Work out the finished part from the listing and answer in its coordinate system (mm). A direction names the side the tool comes from. Coordinates: 2 decimals unless noted, no trailing zeros. Write each loop counter-clockwise with the first axis right and the second up, starting at its lowest first coordinate (ties: lowest second). Pieces come first, ordered by that corner, then holes. Notation, with made-up numbers: M -29.75,84 L -13.75,84 A16 ccw -13.75,107 Z; hole C 31.25,-16.5 d6. An arc over 180 degrees is marked long. Answer as CSV lines item,"result". Start each with the question number.
(1) The mould has two halves that part along Y. Classify faces 1 (the flat face through (10, -4, 7)), 2 (the flat face through (0, -5, 7)), 3 (the cylindrical face through (4.991, 2.123, 7.395)), 4 (the cylindrical face through (-14.991, 2.123, 7.395)): released by +Y, released by -Y, zero draft, split by the parting line, or undercut.
(2) A cutting plane is placed at A-A on x = 2.5. Give the vertices of the cut face in (y, z).
(3) A cutting plane is placed at D-D on x = -17.5. Give the vertices of the cut face in (y, z), then the cut area to 3 significant figures.
(4) Flat-ended cylindrical pins translate along their axes: P1, Ø1.5, axis at y = -1, z = 3, coming from the -X side; P2, Ø3, axis at y = 4, z = 4.5, coming from the -X side; P3, Ø1, axis at x = -13.5, z = 4, coming from the -Y side. Find the tip coordinate at first contact, or state that the pin passes through.
(5) Find the intervals of material crossed by L1, parallel to Y at x = 2.5, z = 7.5; L2, parallel to Y at x = 5, z = 9; L3, parallel to X at y = -4, z = 1, in increasing order. Write a range as [from, to].
(6) For faces 5 (the cylindrical face through (7.6, -3, 7.4)), 6 (the flat face through (-10, 4, 7)), 7 (the flat face through (-5, 0, 0)), 8 (the flat face through (10, 4, 7)), 9 (the flat face through (-10, -4, 7)), determine the directions among +Z, -Z, +X, -X, +Y, -Y from which every point of the face is accessible in a straight line to the end or side of a thin tool.
(7) A cutting plane is placed at C-C on y = 0. Give the vertices of the cut face in (x, z), then the cut area to 3 significant figures.
(8) A cutting plane is placed at B-B on z = 8.5. Give the vertices of the cut face in (x, y) (1 decimal).
from build123d import *

# Parameters (mm, degrees)
F1_DEPTH = 15


with BuildPart() as f1:
    # F0 (on Top) → F1 (new body)
    with BuildSketch(Plane.XY):
        with BuildLine():
            Line((-10, -5), (10, -5))
            Line((10, -5), (10, -2.459675))
            ThreePointArc((10, -2.459675), (9.822474, -2.185813), (9.5, -2.236068))
            ThreePointArc((9.5, -2.236068), (7.581884, -2.998882), (5.625, -2.341874))
            ThreePointArc((5.625, -2.341874), (5, -2.122499), (4.375, -2.341874))
            ThreePointArc((4.375, -2.341874), (-0.5, 0), (4.375, 2.341874))
            ThreePointArc((4.375, 2.341874), (5, 2.122499), (5.625, 2.341874))
            ThreePointArc((5.625, 2.341874), (7.581884, 2.998882), (9.5, 2.236068))
            ThreePointArc((9.5, 2.236068), (9.822474, 2.185813), (10, 2.459675))
            Line((10, 2.459675), (10, 5))
            Line((10, 5), (-10, 5))
            Line((-10, 5), (-10, 2.459675))
            ThreePointArc((-10, 2.459675), (-10.177526, 2.185813), (-10.5, 2.236068))
            ThreePointArc((-10.5, 2.236068), (-12.418116, 2.998882), (-14.375, 2.341874))
            ThreePointArc((-14.375, 2.341874), (-15, 2.122499), (-15.625, 2.341874))
            ThreePointArc((-15.625, 2.341874), (-20.5, 0), (-15.625, -2.341874))
            ThreePointArc((-15.625, -2.341874), (-15, -2.122499), (-14.375, -2.341874))
            ThreePointArc((-14.375, -2.341874), (-12.418116, -2.998882), (-10.5, -2.236068))
            ThreePointArc((-10.5, -2.236068), (-10.177526, -2.185813), (-10, -2.459675))
            Line((-10, -2.459675), (-10, -5))
        make_face()
    extrude(amount=F1_DEPTH)


solid = f1.part
Here are the results:
1,face 1,"zero draft"
1,face 2,"released by -Y"
1,face 3,"undercut"
1,face 4,"released by +Y"
2,outline,"M -5,0 L -3,0 L -3,15 L -5,15 Z; M 3,0 L 5,0 L 5,15 L 3,15 Z"
3,outline,"M -3,0 L 3,0 L 3,15 L -3,15 Z"
3,area,"90.0 mm^2"
4,P1,"stops at x = -20.49"
4,P2,"stops at x = -19.16"
4,P3,"stops at y = -2.96"
5,L1,"y = [-5, -3], [3, 5]"
5,L2,"y = [-5, -2.12], [2.12, 5]"
5,L3,"x = [-10, 10]"
6,face 5,"+Z, -Z"
6,face 6,"+Z, -Z, +Y"
6,face 7,"-Z, +X, -X, +Y, -Y"
6,face 8,"+Z, -Z, +X, +Y, -Y"
6,face 9,"+Z, -Z, -Y"
7,outline,"M -20.5,0 L -0.5,0 L -0.5,15 L -20.5,15 Z"
7,area,"300 mm^2"
8,outline,"M -15.6,-2.3 A1 cw -14.4,-2.3 A3 ccw -10.5,-2.2 A0.3 cw -10,-2.5 L -10,-5 L 10,-5 L 10,-2.5 A0.3 ccw 9.5,-2.2 A3 cw 5.6,-2.3 A1 ccw 4.4,-2.3 A3 cw long 4.4,2.3 A1 ccw 5.6,2.3 A3 cw 9.5,2.2 A0.3 ccw 10,2.5 L 10,5 L -10,5 L -10,2.5 A0.3 cw -10.5,2.2 A3 ccw -14.4,2.3 A1 cw -15.6,2.3 A3 ccw long Z"
